Check sheet for the modelled part. Datum: model origin and axes. Units: mm. A direction names the side the tool comes from. Give positions to 0.01 mm unless a question says otherwise; leave off trailing zeros. Loops run counter-clockwise (first coordinate to the right, second up) from the corner with the lowest first, then second, coordinate; pieces in that order, holes last.
```python
from build123d import *

# Parameters (mm, degrees)
SKETCH1_R           = 4.25
BOSS_EXTRUDE1_DEPTH = 15
SKETCH3_R           = 8.25
CUT_EXTRUDE1_DEPTH  = 46.05
SKETCH4_R           = 5
CUT_EXTRUDE3_DEPTH  = 46.05
SKETCH5_R           = 3.5
CUT_EXTRUDE4_DEPTH  = 46.05
BOSS_EXTRUDE2_DEPTH = 9
FILLET1_R           = 13


with BuildPart() as part:
    # Sketch1 → Boss-Extrude1 (new body)
    with BuildSketch(Plane.XY):
        with BuildLine():
            Line((-8.1, 22.5), (-8.1, 129.9))
            Line((-8.1, 129.9), (0.9, 129.9))
            Line((0.9, 129.9), (0.9, 35.5))
            ThreePointArc((0.9, 35.5), (4.707611845, 26.307611845), (13.9, 22.5))
            Line((13.9, 22.5), (20.5, 22.5))
            Line((20.5, 22.5), (20.5, -22.5))
            Line((20.5, -22.5), (-26.3, -22.5))
            Line((-26.3, -22.5), (-26.3, 22.5))
            Line((-26.3, 22.5), (-8.1, 22.5))
        make_face()
        with Locations((-11.95, -14.95)):
            Circle(SKETCH1_R, mode=Mode.SUBTRACT)
        with Locations((11.95, -14.95)):
            Circle(SKETCH1_R, mode=Mode.SUBTRACT)
        with Locations((11.95, 14.95)):
            Circle(SKETCH1_R, mode=Mode.SUBTRACT)
        with Locations((-11.95, 14.95)):
            Circle(SKETCH1_R, mode=Mode.SUBTRACT)
    extrude(amount=BOSS_EXTRUDE1_DEPTH)

    # Sketch3 → Cut-Extrude1 (cut)
    with BuildSketch(Plane.ZY.offset(26.3)):
        with Locations((14.5, 0)):
            Circle(SKETCH3_R)
    extrude(amount=-CUT_EXTRUDE1_DEPTH, mode=Mode.SUBTRACT)

    # Sketch4 → Cut-Extrude3 (cut)
    with BuildSketch(Plane(origin=(0.9, 0, 0), x_dir=(0, 0, -1), z_dir=(1, 0, 0))):
        with Locations((-7.5, 86.9)):
            Circle(SKETCH4_R)
        with Locations((-7.5, 114.9)):
            Circle(SKETCH4_R)
    extrude(amount=-CUT_EXTRUDE3_DEPTH, mode=Mode.SUBTRACT)

    # Sketch5 → Cut-Extrude4 (cut)
    with BuildSketch(Plane(origin=(20.5, 0, 0), x_dir=(0, 0, -1), z_dir=(1, 0, 0))):
        with Locations((-15, 0)):
            Circle(SKETCH5_R)
    extrude(amount=-CUT_EXTRUDE4_DEPTH, mode=Mode.SUBTRACT)

    # Sketch6 → Boss-Extrude2 (add)
    with BuildSketch(Plane.ZY.offset(8.1)):
        with BuildLine():
            Line((15, 76.386851455), (18.651630299, 84.554112306))
            ThreePointArc((18.651630299, 84.554112306), (18.911938215, 85.352068488), (19, 86.186777661))
            Line((19, 86.186777661), (19, 120.550049196))
            ThreePointArc((19, 120.550049196), (18.902685036, 121.427003874), (18.615475246, 122.261288146))
            Line((18.615475246, 122.261288146), (15, 129.9))
            Line((15, 129.9), (15, 76.386851455))
        make_face()
        with BuildLine():
            Line((-3.615475246, 122.261288146), (0, 129.9))
            Line((0, 129.9), (0, 76.386851455))
            Line((0, 76.386851455), (-3.651630299, 84.554112306))
            ThreePointArc((-3.651630299, 84.554112306), (-3.911938215, 85.352068488), (-4, 86.186777661))
            Line((-4, 86.186777661), (-4, 120.550049196))
            ThreePointArc((-4, 120.550049196), (-3.902685036, 121.427003874), (-3.615475246, 122.261288146))
        make_face()
    extrude(amount=-BOSS_EXTRUDE2_DEPTH)

    # Fillet1
    fillet1_edges = [part.edges().sort_by_distance(p)[0] for p in [
        (-8.1, 22.5, 7.5),
    ]]
    fillet(fillet1_edges, radius=FILLET1_R)


solid = part.part
```
(1) Gauge pin test, flat ends, axial feed: pin 1 Ø13.5 at (x, y) = (11.95, -14.95) entering from -Z; pin 2 Ø13.5 at (x, y) = (-11.95, 14.95) entering from +Z; pin 3 Ø7 at (y, z) = (4, 8.5) entering from -X; pin 4 Ø2 at (y, z) = (51, 13) entering from -X. Record the tip position at first contact, or that the pin passes through.
(2) Section check A-A on y = 14.95. Record the boundary of the cut face in (x, z), plus the area to 3 significant figures.
(3) Section check B-B on x = 12. Record the boundary of the cut face in (y, z), plus the area to 3 significant figures.
(4) Section check C-C on y = 44.5. Record the boundary of the cut face in (x, z), plus the area to 3 significant figures.
(5) Section check D-D on x = -11.95. Record the boundary of the cut face in (y, z), plus the area to 3 significant figures.
(6) Material ranges on line 1 (Z direction, x = -4, y = 86); line 2 (Y direction, x = 17.5, z = 12); line 3 (Y direction, x = -5.5, z = 7.5), recorded low to high.
(7) Access from +Z, -Z, +X, -X, +Y, -Y to the whole of each face (thin tool, end or side, straight path). Record for faces 1 (the face through (19.75, 0, 11)), 2 (the face through (-3, 32, 15)), 3 (the face through (-8.1, 83, 2)).
(8) Release check for a two-part mould opening along Y. For faces 4 (the face through (-24, 22.5, 7)), 5 (the face through (-4, 103, -4)), 6 (the face through (-3.537, 91.116, 4.812)) record: pulls with the +Y half, pulls with the -Y half, needs draft (parallel to the pull), parting line crosses it, or undercut.
Computed values:
1. pin 1: stops at z = 0
1. pin 2: stops at z = 15
1. pin 3: stops at x = -26.3
1. pin 4: stops at x = -8.1
2. outline: (-26.3, 0) - (-16.2, 0) - (-16.2, 15) - (-26.3, 15) - close; (-7.7, 0) - (7.7, 0) - (7.7, 15) - (-7.7, 15) - close; (16.2, 0) - (20.5, 0) - (20.5, 15) - (16.2, 15) - close
2. area: 447 mm2
3. outline: (-22.5, 0) - (-19.2, 0) - (-19.2, 15) - (-22.5, 15) - close; (-10.7, 0) - (10.7, 0) - (10.7, 15) - (8.23, 15) arc R8.25 cw (long way) to (-8.23, 15) - (-10.7, 15) - close; (19.2, 0) - (22.64, 0) - (22.64, 15) - (19.2, 15) - close
3. area: 307 mm2
4. outline: (-8.1, 0) - (0.9, 0) - (0.9, 15) - (-8.1, 15) - close
4. area: 135 mm2
5. outline: (-22.5, 0) - (-19.2, 0) - (-19.2, 15) - (-22.5, 15) - close; (-10.7, 0) - (10.7, 0) - (10.7, 15) - (8.23, 15) arc R8.25 cw (long way) to (-8.23, 15) - (-10.7, 15) - close; (19.2, 0) - (26.27, 0) - (26.27, 15) - (19.2, 15) - close
5. area: 361 mm2
6. line 1: z = -4 to 2.58, 12.42 to 19
6. line 2: y = -22.5 to -7.86, 7.86 to 22.5
6. line 3: y = -22.5 to -4.37, 4.37 to 81.9, 91.9 to 109.9, 119.9 to 129.9
7. face 1: +Z, -X
7. face 2: +Z, +X, -X, -Y
7. face 3: +Z, -Z, -X, +Y
8. face 4: pulls with the +Y half
8. face 5: needs draft
8. face 6: undercut
